```python
from build123d import *

# Parameters (mm, degrees)
SKETCH2_W           = 15.24
SKETCH2_H           = 20.32
BOSS_EXTRUDE4_DEPTH = 2.159
EXTRUDE_THIN2_DEPTH = 40.64


with BuildPart() as part:
    # Sketch2 → Boss-Extrude4 (new body)
    with BuildSketch(Plane.XY):
        with BuildLine():
            Line((166.65702, 132.382444359), (166.65702, 93.98))
            Line((166.65702, 93.98), (200.94702, 93.98))
            Line((200.94702, 93.98), (207.037726035, 102.87))
            Line((207.037726035, 102.87), (254.512766428, 102.87))
            Line((254.512766428, 102.87), (260.603472462, 93.98))
            Line((260.603472462, 93.98), (294.893472462, 93.98))
            Line((294.893472462, 93.98), (294.893472462, 132.382444359))
            ThreePointArc((294.893472462, 132.382444359), (230.775246231, 156.110938615), (166.65702, 132.382444359))
        make_face()
        with Locations((252.365246231, 126.944020361)):
            Rectangle(SKETCH2_W, SKETCH2_H, mode=Mode.SUBTRACT)
        with Locations((209.185246231, 126.944020361)):
            Rectangle(SKETCH2_W, SKETCH2_H, mode=Mode.SUBTRACT)
        with Locations((230.775246231, 126.944020361)):
            Rectangle(SKETCH2_W, SKETCH2_H, mode=Mode.SUBTRACT)
    extrude(amount=BOSS_EXTRUDE4_DEPTH)

    # Sketch2<7> → Extrude-Thin2 (add)
    with BuildSketch(Plane.XY):
        with BuildLine():
            Line((164.11702, 133.541292), (164.11702, 91.44))
            Line((164.11702, 91.44), (202.285763232, 91.44))
            Line((202.285763232, 91.44), (208.376469266, 100.33))
            Line((208.376469266, 100.33), (253.174023196, 100.33))
            Line((253.174023196, 100.33), (259.264729231, 91.44))
            Line((259.264729231, 91.44), (297.433472462, 91.44))
            Line((297.433472462, 91.44), (297.433472462, 133.541292))
            ThreePointArc((297.433472462, 133.541292), (230.775246231, 158.650938615), (164.11702, 133.541292))
        make_face()
        with BuildLine():
            Line((166.65702, 132.382444359), (166.65702, 93.98))
            Line((166.65702, 93.98), (200.94702, 93.98))
            Line((200.94702, 93.98), (207.037726035, 102.87))
            Line((207.037726035, 102.87), (254.512766428, 102.87))
            Line((254.512766428, 102.87), (260.603472462, 93.98))
            Line((260.603472462, 93.98), (294.893472462, 93.98))
            Line((294.893472462, 93.98), (294.893472462, 132.382444359))
            ThreePointArc((294.893472462, 132.382444359), (230.775246231, 156.110938615), (166.65702, 132.382444359))
        make_face(mode=Mode.SUBTRACT)
    extrude(amount=EXTRUDE_THIN2_DEPTH)


solid = part.part
```
The listing builds one solid part. Answer for the finished solid, in the listing's coordinates (mm). A direction names the side the tool comes from. Coordinates: 2 decimals unless noted, no trailing zeros. Write each loop counter-clockwise with the first axis right and the second up, starting at its lowest first coordinate (ties: lowest second). Pieces come first, ordered by that corner, then holes. Notation, with made-up numbers: (-12, -7) - (42, -7) arc R18 cw to (42, 19) - close; hole circle Ø5 at (10.25, -37.5). An arc over 180 degrees is marked (long way). Return JSON: item names as keys, results as strings. Group by question number.
1. A cutting plane is placed at C-C, the plane x = 256. Determine the outline of the cut face in (y, z).
2. A cutting plane is placed at D-D, the plane y = 141.5. Determine the outline of the cut face in (x, z), plus the area to 3 significant figures.
3. Which of the six approach directions +Z, -Z, +X, -X, +Y, -Y give full straight-line access (tool end or side, diameter ignored) to faces 5 (the flat face through (230, 112, 2.159)), 6 (the flat face through (183, 91.44, 20)), 7 (the flat face through (205.288, 95.823, 20.036))?
4. Determine the mould class of faces 1 (the flat face through (278, 93.98, 21)), 2 (the cylindrical face through (231.794, 158.646, 20.036)), 3 (the flat face through (166.657, 113, 21)), 4 (the flat face through (230, 111, 0)) for opening direction X: released by +X, released by -X, zero draft, split by the parting line, or undercut.
5. A cutting plane is placed at A-A, the plane y = 124. Determine the outline of the cut face in (x, z).
6. A cutting plane is placed at B-B, the plane z = 9. Determine the outline of the cut face in (x, y).
7. Straight lines are drawn through the part: L1, parallel to X at y = 109, z = 38; L2, parallel to X at y = 96, z = 2.5; L3, parallel to X at y = 102, z = 17.5. For each, find the intervals that lie inside material, in ascending order.
8. Given pin 1 (2.5 mm diameter, centred on x = 210.5, z = 1, fed in from -Y); pin 2 (1 mm diameter, centred on y = 145.5, z = 13.5, fed in from -X); pin 3 (1.1 mm diameter, centred on x = 213, z = 1, fed in from +Y), each flat-ended and moving along its own axis, determine where each tip first touches the part or whether it passes through.
Ans:
{
 "1": {"outline": "(96.21, 0) - (116.78, 0) - (116.78, 2.16) - (100.7, 2.16) - (100.7, 40.64) - (96.21, 40.64) - close; (137.1, 0) - (155.45, 0) - (155.45, 40.64) - (152.83, 40.64) - (152.83, 2.16) - (137.1, 2.16) - close"},
 "2": {"outline": "(174.46, 0) - (287.09, 0) - (287.09, 40.64) - (282.4, 40.64) - (282.4, 2.16) - (179.15, 2.16) - (179.15, 40.64) - (174.46, 40.64) - close", "area": "605 mm²"},
 "3": {"face 5": "+Z", "face 6": "+Z, -Z, +X, -X, -Y", "face 7": "+Z, -Z, -Y"},
 "4": {"face 1": "undercut", "face 2": "split by the parting line", "face 3": "undercut", "face 4": "zero draft"},
 "5": {"outline": "(164.12, 0) - (201.57, 0) - (201.57, 2.16) - (166.66, 2.16) - (166.66, 40.64) - (164.12, 40.64) - close; (216.81, 0) - (223.16, 0) - (223.16, 2.16) - (216.81, 2.16) - close; (238.4, 0) - (244.75, 0) - (244.75, 2.16) - (238.4, 2.16) - close; (259.99, 0) - (297.43, 0) - (297.43, 40.64) - (294.89, 40.64) - (294.89, 2.16) - (259.99, 2.16) - close"},
 "6": {"outline": "(164.12, 91.44) - (202.29, 91.44) - (208.38, 100.33) - (253.17, 100.33) - (259.26, 91.44) - (297.43, 91.44) - (297.43, 133.54) arc R101.03 ccw to (164.12, 133.54) - close; hole (166.66, 93.98) - (200.95, 93.98) - (207.04, 102.87) - (254.51, 102.87) - (260.6, 93.98) - (294.89, 93.98) - (294.89, 132.38) arc R98.49 ccw to (166.66, 132.38) - close"},
 "7": {"L1": "164.12 to 166.66, 294.89 to 297.43", "L2": "164.12 to 166.66, 202.33 to 205.41, 256.14 to 259.22, 294.89 to 297.43", "L3": "164.12 to 166.66, 206.44 to 255.11, 294.89 to 297.43"},
 "8": {"pin 1": "y = 100.33", "pin 2": "x = 180.06", "pin 3": "y = 157.17"}
}
